from build123d import *

# Parameters (mm, degrees)
SKETCH1_W           = 47
SKETCH1_H           = 40
SKETCH1_R           = 1.75
BOSS_EXTRUDE1_DEPTH = 3
SKETCH2_W           = 10
SKETCH2_H           = 10
BOSS_EXTRUDE3_DEPTH = 27
SKETCH3_W           = 45
SKETCH3_H           = 10
SKETCH3_W_2         = 10
BOSS_EXTRUDE4_DEPTH = 6
SKETCH4_W           = 55
SKETCH4_H           = 10
CUT_EXTRUDE1_DEPTH  = 6
SKETCH5_W           = 55
SKETCH5_H           = 10
BOSS_EXTRUDE5_DEPTH = 6
SKETCH6_R           = 2.5
CUT_EXTRUDE2_DEPTH  = 92.094730912


with BuildPart() as part:
    # Sketch1 → Boss-Extrude1 (new body)
    with BuildSketch(Plane(origin=(0, 0, 0), x_dir=(1, 0, 0), z_dir=(0, 1, 0))):
        with Locations((23.5, 20)):
            Rectangle(SKETCH1_W, SKETCH1_H)
        with Locations(Location((2.3, 2.9, 0), (0, 0, 270))):
            Circle(SKETCH1_R, mode=Mode.SUBTRACT)
        with Locations(Location((2.3, 37.1, 0), (0, 0, 270))):
            Circle(SKETCH1_R, mode=Mode.SUBTRACT)
        with Locations(Location((39.7, 32.7, 0), (0, 0, 270))):
            Circle(SKETCH1_R, mode=Mode.SUBTRACT)
        with Locations(Location((39.7, 7.3, 0), (0, 0, 270))):
            Circle(SKETCH1_R, mode=Mode.SUBTRACT)
    extrude(amount=BOSS_EXTRUDE1_DEPTH)

    # Sketch2 → Boss-Extrude3 (add)
    with BuildSketch(Plane(origin=(0, 3, 0), x_dir=(1, 0, 0), z_dir=(0, 1, 0))):
        with Locations((23.5, 20)):
            Rectangle(SKETCH2_W, SKETCH2_H)
    extrude(amount=BOSS_EXTRUDE3_DEPTH)

    # Sketch3 → Boss-Extrude4 (add)
    with BuildSketch(Plane(origin=(0, 30, 0), x_dir=(1, 0, 0), z_dir=(0, 1, 0))):
        with Locations((51, 20)):
            Rectangle(SKETCH3_W, SKETCH3_H)
        with Locations((23.5, 20)):
            Rectangle(SKETCH3_W_2, SKETCH3_H)
    extrude(amount=BOSS_EXTRUDE4_DEPTH)

    # Sketch4 → Cut-Extrude1 (cut)
    with BuildSketch(Plane(origin=(0, 36, 0), x_dir=(1, 0, 0), z_dir=(0, 1, 0))):
        with Locations((46, 20)):
            Rectangle(SKETCH4_W, SKETCH4_H)
    extrude(amount=-CUT_EXTRUDE1_DEPTH, mode=Mode.SUBTRACT)

    # Sketch5 → Boss-Extrude5 (add)
    with BuildSketch(Plane(origin=(0, 30, 0), x_dir=(1, 0, 0), z_dir=(0, 1, 0))):
        with Locations((46, 20)):
            Rectangle(SKETCH5_W, SKETCH5_H)
    extrude(amount=BOSS_EXTRUDE5_DEPTH)

    # Sketch6 → Cut-Extrude2 (cut, through all)
    with BuildSketch(Plane(origin=(0, 36, 0), x_dir=(1, 0, 0), z_dir=(0, 1, 0))):
        with Locations(Location((68.5, 20, 0), (0, 0, 270))):
            Circle(SKETCH6_R)
        with Locations(Location((61.5, 20, 0), (0, 0, 270))):
            Circle(SKETCH6_R)
        with Locations(Location((54.5, 20, 0), (0, 0, 270))):
            Circle(SKETCH6_R)
    extrude(amount=-CUT_EXTRUDE2_DEPTH, mode=Mode.SUBTRACT)


solid = part.part
Verification items for the finished model (mm, model axes). A direction names the side the tool comes from. Give positions to 0.01 mm unless a question says otherwise; leave off trailing zeros. Loops run counter-clockwise (first coordinate to the right, second up) from the corner with the lowest first, then second, coordinate; pieces in that order, holes last.
1. Release check for a two-part mould opening along Z. For faces 1 (the flat face through (46, 36, -20)), 2 (the flat face through (23, 1, -40)), 3 (the cylindrical face through (54.6, 33, -22.5)), 4 (the cylindrical face through (2.38, 1.48, -38.85)) record: +Z half, -Z half, draft (parallel to the pull), parting line (faces both ways), or undercut.
Derived:
face 1: draft
face 2: -Z half
face 3: undercut
face 4: undercut
2. Cross-section at D-D on x = 39.7. Record the cut outline in (y, z), and give its area (3 significant figures).
Derived:
outline: (0, -40) - (3, -40) - (3, -34.45) - (0, -34.45) - close; (0, -30.95) - (3, -30.95) - (3, -9.05) - (0, -9.05) - close; (0, -5.55) - (3, -5.55) - (3, 0) - (0, 0) - close; (30, -25) - (36, -25) - (36, -15) - (30, -15) - close
area: 159 mm2
3. Cross-section at B-B on z = -20. Record the cut outline in (x, y), and give its area (3 significant figures).
Derived:
outline: (0, 0) - (47, 0) - (47, 3) - (28.5, 3) - (28.5, 30) - (52, 30) - (52, 36) - (18.5, 36) - (18.5, 3) - (0, 3) - close; (57, 30) - (59, 30) - (59, 36) - (57, 36) - close; (64, 30) - (66, 30) - (66, 36) - (64, 36) - close; (71, 30) - (73.5, 30) - (73.5, 36) - (71, 36) - close
area: 651 mm2
4. Tool access check on faces 5 (the flat face through (33.4, 30.3, -15)), 6 (the flat face through (47, 1, -20)), 7 (the flat face through (51, 30, -20)), 8 (the flat face through (18.5, 19, -20)). Record the directions out of +Z, -Z, +X, -X, +Y, -Y that give a thin tool (end or side, any length) a straight path to the whole face; none if there is none.
Derived:
face 5: +Z, +X, -X, +Y
face 6: +Z, -Z, +X, -Y
face 7: +Z, -Z, +X
face 8: +Z, -Z, -X, +Y
5. Material ranges on probe 1 along X at (y, z) = (31, -20); probe 2 along X at (y, z) = (1.1, -7.3); probe 3 along Y at (x, z) = (42, -17.5), recorded low to high.
Derived:
probe 1: x = 18.5 to 52, 57 to 59, 64 to 66, 71 to 73.5
probe 2: x = 0 to 37.95, 41.45 to 47
probe 3: y = 0 to 3, 30 to 36
6. Cross-section at C-C on z = -32.7. Record the cut outline in (x, y).
Derived:
outline: (0, 0) - (37.95, 0) - (37.95, 3) - (0, 3) - close; (41.45, 0) - (47, 0) - (47, 3) - (41.45, 3) - close
7. Go/stop test with flat-tipped pins: P1, Ø10, axis at x = 36.5, y = 14.5, coming from the +Z side; P2, Ø3, axis at y = 18.5, z = -22, coming from the -X side; P3, Ø11, axis at y = 11, z = -19, coming from the +X side; P4, Ø3.5, axis at y = 1.5, z = -21.5, coming from the +X side. Record where each tip stops, or that it passes through.
Derived:
P1: passes through
P2: stops at x = 18.5
P3: stops at x = 28.5
P4: stops at x = 47
8. Cross-section at A-A on x = 54.5. Record the cut outline in (y, z).
Derived:
outline: (30, -25) - (36, -25) - (36, -22.5) - (30, -22.5) - close; (30, -17.5) - (36, -17.5) - (36, -15) - (30, -15) - close
